Geometry: final body of the model. Coordinates: model frame, mm. A direction names the side the tool comes from. Coordinates: 2 decimals unless noted, no trailing zeros. Loops run counter-clockwise (first coordinate to the right, second up) from the corner with the lowest first, then second, coordinate; pieces in that order, holes last. Notation, with made-up numbers: (48, 41.5) - (67, 41.5) arc R19 ccw to (67, 78.5) - close; hole circle Ø4 at (-9.5, -28). An arc over 180 degrees is marked (long way). Put each result on its own line as item: value. Start each with the question number.
1) Material intervals for line 1 along Y through (x, z) = (58.5, 3.5); line 2 along X through (y, z) = (26, 11.5); line 3 along Y through (x, z) = (-62.5, 2.5), sorted ascending. Write a range as from..to.
2) Reachability of faces 4 (the cylindrical face through (-41.67, 16.32, 7.16)), 5 (the cylindrical face through (34.73, -17.9, 9.57)), 6 (the flat face through (-42.164, -4, 7)) from +Z, -Z, +X, -X, +Y, -Y: full face, straight path, thin tool, end or side. Return the list, or none.
3) Draft query along Y for faces 1 (the cylindrical face through (24.385, 9.491, 7.163)), 2 (the flat face through (66.63, 28.62, 3.13)), 3 (the flat face through (35.814, 8, 9)). Return one class per face: +Y half, -Y half, draft (parallel to the pull), parting line (faces both ways), or undercut.
4) Section B-B on z = 7.75. Output: boundary loops of the cut face in (x, y).
5) Section A-A on y = 21. Output: boundary loops of the cut face in (x, z) (3 decimals).
6) Section D-D on y = 6.5. Output: boundary loops of the cut face in (x, z) (3 decimals).
7) Section C-C on x = 38. Output: boundary loops of the cut face in (y, z).
8) Contact query for flat-ended pins moving along their axis: pin 1 Ø5 at (y, z) = (-5, 5.5) entering from -X; pin 2 Ø5.5 at (x, z) = (-21.5, 5.5) entering from +Y; pin 3 Ø3 at (y, z) = (10.5, 9) entering from -X. Output: stop coordinate, or through.
```python
from build123d import *

# Parameters (mm, degrees)
F0_R     = 1.7145
F0_R_2   = 1.27
F1_DEPTH = 6.35
F2_W     = 120.65
F2_H     = 51.054
F3_DEPTH = 1.778
F4_R     = 1.27
F5_DEPTH = 6.35
F6_SIZE  = 6.35
F7_R     = 3.81
F8_SIZE  = 1.27


# Not quite as in the source:
# - a feature names something its author has since deleted; it is built from what else it names


with BuildPart() as f1:
    # F0 (on Top) → F1 (new body)
    with BuildSketch(Plane.XY):
        with BuildLine():
            Line((69.85, -31.75), (69.85, 31.75))
            Line((69.85, 31.75), (29.464, 31.75))
            Line((29.464, 31.75), (29.464, 15.6197039467))
            ThreePointArc((29.464, 15.6197039467), (24.384, 9.398), (29.464, 3.1762960533))
            Line((29.464, 3.1762960533), (29.464, -12.7))
            Line((29.464, -12.7), (-42.164, -12.7))
            Line((-42.164, -12.7), (-42.164, 3.1762960533))
            ThreePointArc((-42.164, 3.1762960533), (-37.084, 9.398), (-42.164, 15.6197039467))
            Line((-42.164, 15.6197039467), (-42.164, 31.75))
            Line((-42.164, 31.75), (-69.85, 31.75))
            Line((-69.85, 31.75), (-69.85, 22.86))
            Line((-69.85, 22.86), (-50.8, 22.86))
            Line((-50.8, 22.86), (-50.8, -22.86))
            Line((-50.8, -22.86), (-69.85, -22.86))
            Line((-69.85, -22.86), (-69.85, -31.75))
            Line((-69.85, -31.75), (69.85, -31.75))
        make_face()
        with Locations((-57.404, -27.178)):
            Circle(F0_R, mode=Mode.SUBTRACT)
        with Locations((57.404, -27.178)):
            Circle(F0_R, mode=Mode.SUBTRACT)
        with Locations((-43.434, 9.398)):
            Circle(F0_R_2, mode=Mode.SUBTRACT)
        with Locations((-57.404, 27.178)):
            Circle(F0_R, mode=Mode.SUBTRACT)
        with Locations((30.734, 9.398)):
            Circle(F0_R_2, mode=Mode.SUBTRACT)
        with Locations((57.404, 27.178)):
            Circle(F0_R, mode=Mode.SUBTRACT)
    extrude(amount=F1_DEPTH)

    # F2 (on Top) → F3 (cut)
    with BuildSketch(Plane.XY):
        Rectangle(F2_W, F2_H)
    extrude(amount=F3_DEPTH, mode=Mode.SUBTRACT)

    # F4 (on face) → F5 (join)
    with BuildSketch(Plane.XY.offset(6.35)):
        with BuildLine():
            Line((-48.514, 31.75), (-48.514, -19.05))
            Line((-48.514, -19.05), (35.814, -19.05))
            Line((35.814, -19.05), (35.814, 31.75))
            Line((35.814, 31.75), (29.464, 31.75))
            Line((29.464, 31.75), (29.464, 15.6197039467))
            ThreePointArc((29.464, 15.6197039467), (24.384, 9.398), (29.464, 3.1762960533))
            Line((29.464, 3.1762960533), (29.464, -12.7))
            Line((29.464, -12.7), (-42.164, -12.7))
            Line((-42.164, -12.7), (-42.164, 3.1762960533))
            ThreePointArc((-42.164, 3.1762960533), (-37.084, 9.398), (-42.164, 15.6197039467))
            Line((-42.164, 15.6197039467), (-42.164, 31.75))
            Line((-42.164, 31.75), (-48.514, 31.75))
        make_face()
        with Locations((-43.434, 9.398)):
            Circle(F4_R, mode=Mode.SUBTRACT)
        with Locations((30.734, 9.398)):
            Circle(F4_R, mode=Mode.SUBTRACT)
    extrude(amount=F5_DEPTH)

    # F6
    f6_edges = [f1.edges().sort_by_distance(p)[0] for p in [
        (-69.85, 31.75, 3.175),
        (69.85, 31.75, 3.175),
        (69.85, -31.75, 3.175),
        (-69.85, -31.75, 3.175),
    ]]
    chamfer(f6_edges, length=F6_SIZE)

    # F7
    f7_edges = [f1.edges().sort_by_distance(p)[0] for p in [
        (-50.8, 22.86, 4.064),
        (-50.8, -22.86, 4.064),
        (29.464, -12.7, 7.239),
        (-42.164, -12.7, 7.239),
        (29.464, 3.176296, 7.239),
        (29.464, 15.619704, 7.239),
        (-42.164, 15.619704, 7.239),
        (-42.164, 3.176296, 7.239),
        (-48.514, -19.05, 9.525),
        (35.814, -19.05, 9.525),
    ]]
    fillet(f7_edges, radius=F7_R)

    # F8
    f8_edges = [f1.edges().sort_by_distance(p)[0] for p in [
        (-59.1185, -27.178, 6.35),
        (-59.1185, 27.178, 6.35),
        (55.6895, 27.178, 6.35),
        (55.6895, -27.178, 6.35),
    ]]
    chamfer(f8_edges, length=F8_SIZE)


solid = f1.part
```
Answer block:
1. line 1: y = -31.75..-28.5, -25.86..25.86, 28.5..31.75
1. line 2: x = -48.51..-42.16, 29.46..35.81
1. line 3: y = -31.75..-22.86, 22.86..31.75
2. face 4: +Z, -Z, +Y
2. face 5: +Z, +X, -Y
2. face 6: +Z, -Z
3. face 1: undercut
3. face 2: +Y half
3. face 3: draft
4. outline: (-48.51, -15.24) arc R3.81 ccw to (-44.7, -19.05) - (32, -19.05) arc R3.81 ccw to (35.81, -15.24) - (35.81, 31.75) - (29.46, 31.75) - (29.46, 18.2) arc R3.81 cw to (27.56, 14.9) arc R6.35 ccw to (27.56, 3.9) arc R3.81 cw to (29.46, 0.6) - (29.46, -8.89) arc R3.81 cw to (25.65, -12.7) - (-38.35, -12.7) arc R3.81 cw to (-42.16, -8.89) - (-42.16, 0.6) arc R3.81 cw to (-40.26, 3.9) arc R6.35 ccw to (-40.26, 14.9) arc R3.81 cw to (-42.16, 18.2) - (-42.16, 31.75) - (-48.51, 31.75) - close; hole circle Ø2.54 at (-43.43, 9.4); hole circle Ø2.54 at (30.73, 9.4)
5. outline: (-51.337, 1.778) - (-42.164, 1.778) - (-42.164, 12.7) - (-48.514, 12.7) - (-48.514, 6.35) - (-51.337, 6.35) - close; (29.464, 1.778) - (60.325, 1.778) - (60.325, 0) - (69.85, 0) - (69.85, 6.35) - (35.814, 6.35) - (35.814, 12.7) - (29.464, 12.7) - close
6. outline: (-50.8, 1.778) - (-37.784, 1.778) - (-37.784, 12.7) - (-48.514, 12.7) - (-48.514, 6.35) - (-50.8, 6.35) - close; (25.084, 1.778) - (60.325, 1.778) - (60.325, 0) - (69.85, 0) - (69.85, 6.35) - (35.814, 6.35) - (35.814, 12.7) - (25.084, 12.7) - close
7. outline: (-31.75, 0) - (-25.53, 0) - (-25.53, 1.78) - (25.53, 1.78) - (25.53, 0) - (31.75, 0) - (31.75, 6.35) - (-31.75, 6.35) - close
8. pin 1: stops at x = -50.8
8. pin 2: stops at y = -12.7
8. pin 3: stops at x = -48.51
